The listing builds one solid part. Answer for the finished solid, in the listing's coordinates (mm). Face numbers are marked on the shaded views. A direction names the side the tool comes from. Coordinates: 2 decimals unless noted, no trailing zeros. Loops run counter-clockwise (first coordinate to the right, second up) from the corner with the lowest first, then second, coordinate; pieces in that order, holes last. Notation, with made-up numbers: (-38.5, 45.5) - (-21.5, 45.5) arc R17 ccw to (-21.5, 50.5) - close; hole circle Ø11 at (55, -12). An arc over 180 degrees is marked (long way). Put each result on its own line as item: value.
```python
from build123d import *

# Parameters (mm, degrees)
F0_R         = 1.4
F1_DEPTH     = 2
F3_DEPTH     = 20
F5_DEPTH     = 2
F6_W         = 24.2574699223
F6_H         = 65.0979466736
F7_DEPTH     = 25
F8_R         = 5
F10_DEPTH    = 9
F11_R        = 5
F12_W        = 12
F12_H        = 2
F13_DEPTH    = 3
F14_T1_DEPTH = 24.9128784748
F16_R        = 3.5
F17_DEPTH    = 25


# Not quite as in the source:
# - a fillet or chamfer that OpenCascade refuses, or shapes differently, is made with other operations: its cross-section is extruded or revolved along the edge and cut away or added


with BuildPart() as f1:
    # F0 (on Top) → F1 (new body)
    with BuildSketch(Plane.XY):
        with BuildLine():
            ThreePointArc((22, -4), (24.8284271247, -2.8284271247), (26, 0))
            ThreePointArc((26, 0), (24.8284271247, 2.8284271247), (22, 4))
            ThreePointArc((22, 4), (18, 0), (22, -4))
        make_face()
        with Locations((22, 0)):
            Circle(F0_R, mode=Mode.SUBTRACT)
        with BuildLine():
            ThreePointArc((22, -4), (18, 0), (22, 4))
            Line((22, 4), (19, 4))
            Line((19, 4), (17, 0))
            Line((17, 0), (19, -4))
            Line((19, -4), (22, -4))
        make_face()
    extrude(amount=F1_DEPTH)

    # F2 (on face) → F3 (join)
    with BuildSketch(Plane.XY.offset(2)):
        Polygon((19, 4), (17, 0), (19, -4), (20.1180339887, -4), (18.1180339887, 0), (20.1180339887, 4), align=None)
    extrude(amount=F3_DEPTH)



with BuildPart() as f1b:
    # F0 (on Top) → F1, piece 2 (new body)
    with BuildSketch(Plane.XY):
        with BuildLine():
            ThreePointArc((-4, -22), (0, -26), (4, -22))
            ThreePointArc((4, -22), (0, -18), (-4, -22))
        make_face()
        with Locations((0, -22)):
            Circle(F0_R, mode=Mode.SUBTRACT)
        with BuildLine():
            ThreePointArc((-4, -22), (0, -18), (4, -22))
            Line((4, -22), (4, -19))
            Line((4, -19), (0, -17))
            Line((0, -17), (-4, -19))
            Line((-4, -19), (-4, -22))
        make_face()
    extrude(amount=F1_DEPTH)

    # F2 (on face) → F3, piece 2 (join)
    with BuildSketch(Plane.XY.offset(2)):
        Polygon((4, -19), (0, -17), (-4, -19), (-4, -20.1180339887), (0, -18.1180339887), (4, -20.1180339887), align=None)
    extrude(amount=F3_DEPTH)


with BuildPart() as f1_1:
    add(f1.part)

    add(f1b.part)  # F5 merges F1b
    # F4 (on face) → F5 (join)
    with BuildSketch(Plane.XY.offset(22)):
        Polygon((4, -20.1180339887), (4, -4), (0, -4), (0, -18.1180339887), align=None)
        Polygon((17, 0), (19, 4), (0, 4), (0, -4), (4, -4), (19, -4), align=None)
        Polygon((18.1180339887, 0), (20.1180339887, 4), (19, 4), (17, 0), (19, -4), (20.1180339887, -4), align=None)
    extrude(amount=F5_DEPTH)

    # F6 (on face) → F7 (cut)
    with BuildSketch(Plane.XY.offset(24)):
        with Locations((-12.1287349612, -10.913932696)):
            Rectangle(F6_W, F6_H)
    extrude(amount=-F7_DEPTH, mode=Mode.SUBTRACT)

    # F8
    f8_edges = [f1_1.edges().sort_by_distance(p)[0] for p in [
        (4, -4, 23),
        (2, -18, 22),
        (18, -2, 22),
        (18, 2, 22),
        (19.118034, -2, 24),
        (19.118034, 2, 24),
        (2, -19.118034, 24),
    ]]
    fillet(f8_edges, radius=F8_R)

    # F9 (on face) → F10 (join)
    with BuildSketch(Plane.XY.offset(24)):
        Polygon((0, -10.8508134726), (0, -12.527864045), (4, -14.527864045), (4, -12.8508134726), (0.6708202289, -11.1862235871), align=None)
    extrude(amount=F10_DEPTH)

    # F11
    f11_edges = [f1_1.edges().sort_by_distance(p)[0] for p in [
        (2, -11.850813, 24),
        (2, -13.527864, 24),
    ]]
    fillet(f11_edges, radius=F11_R)

    # F12 (on face) → F13 (join)
    with BuildSketch(Plane.XY.offset(24)):
        with Locations((6, 3)):
            Rectangle(F12_W, F12_H)
    extrude(amount=F13_DEPTH)

    # F14: fillet of radius 5 on 1 edges, made by hand

    # F14_s2 → F14_t1 (cut)
    with BuildSketch(Plane.XZ.offset(-15.4564392374)):
        with BuildLine():
            ThreePointArc((12, 24), (10.1560370926, 26.1833001327), (7.417424305, 27))
            Line((7.417424305, 27), (12, 27))
            Line((12, 27), (12, 24))
        make_face()
    extrude(amount=F14_T1_DEPTH, mode=Mode.SUBTRACT)

    # F15: F1 across face


with BuildPart() as f1_2:
    add(f1_1.part)
    add(f1_1.part.mirror(Plane(origin=(0, -10.4635359507, 20.0753373273), x_dir=(0, -1, 0), z_dir=(-1, 0, 0))))

    # F16 (on face) → F17 (cut)
    with BuildSketch(Plane(origin=(0, 4, 0), x_dir=(-1, 0, 0), z_dir=(0, 1, 0))):
        with Locations((0, 33)):
            Circle(F16_R)
    extrude(amount=-F17_DEPTH, mode=Mode.SUBTRACT)


solid = f1_2.part
```
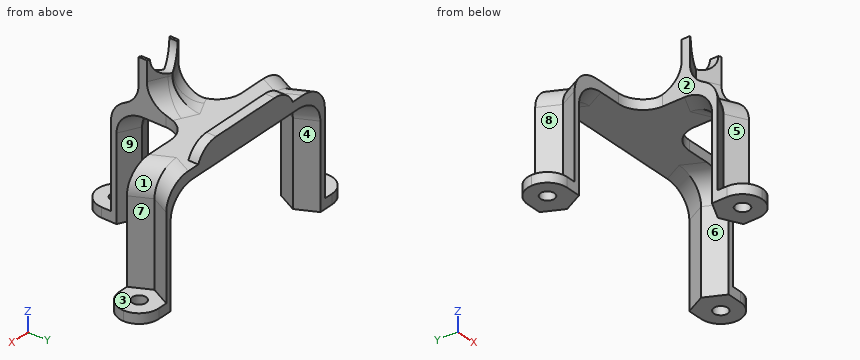
1) The part is cut by section A-A (z = 8). Give the vertices of the cut face in (x, y), and give its area (3 significant figures).
Found:
outline: (-20.12, -4) - (-19, -4) - (-17, 0) - (-19, 4) - (-20.12, 4) - (-18.12, 0) - close; (-4, -20.12) - (0, -18.12) - (4, -20.12) - (4, -19) - (0, -17) - (-4, -19) - close; (17, 0) - (19, -4) - (20.12, -4) - (18.12, 0) - (20.12, 4) - (19, 4) - close
area: 26.8 mm^2
2) The part is cut by section B-B (x = -5.5). Give the vertices of the cut face in (y, z).
Found:
outline: (-5.43, 22) - (4, 22) - (4, 27) - (2, 27) - (2, 24) - (-5.43, 24) - close
3) Straight lines are drawn through the part: L1, parallel to Y at x = 22, z = 1.2; L2, parallel to X at y = -3.25, z = 13.5 (3 decimals); L3, parallel to Z at x = 0, y = 2.5. For each, find the intervals that lie inside material, in ascending order. Write a range as [from, to].
Found:
L1: y = [-4, -1.4], [1.4, 4]
L2: x = [-19.743, -18.625], [18.625, 19.743]
L3: z = [22, 27]
4) The part is cut by section C-C (z = 25.5). Give the vertices of the cut face in (x, y).
Found:
outline: (-10.99, 2) - (10.99, 2) - (10.99, 4) - (-10.99, 4) - close; (-4, -15.08) - (0, -13.08) - (4, -15.08) - (4, -11.25) - (0, -9.25) - (-4, -11.25) - close
5) For a pull along X with two mould halves and no side action, classify the marked faces 1, 2, 3 and 4 as pulls with the +X half, pulls with the -X half, needs draft (parallel to the pull), parting line crosses it, or undercut.
Found:
face 1: pulls with the +X half
face 2: pulls with the -X half
face 3: needs draft
face 4: undercut
6) For the marked faces 5, 6, 7, 8 and 9, determine the directions among +Z, -Z, +X, -X, +Y, -Y from which every point of the face is accessible in a straight line to the end or side of a thin tool.
Found:
face 5: +Z, -Y
face 6: -Z, -Y
face 7: +Z, +X
face 8: +Z, -X
face 9: -Z, +X, +Y
7) Each of these flat-tipped pins is pushed along its axis until it touches: pin 1 (12.5 mm diameter, centred on x = 5.5, y = 0, fed in from +Z); pin 2 (1 mm diameter, centred on y = -22, z = 13, fed in from -X); pin 3 (3 mm diameter, centred on x = -22, y = 0, fed in from +Z); pin 4 (0.9 mm diameter, centred on x = 2.5, z = 26, fed in from -Y). Where does it stop, or does it pass through?
Found:
pin 1: stops at z = 27
pin 2: passes through
pin 3: stops at z = 2
pin 4: stops at y = -14.39
